Can you work these out from the model? Positions are in its coordinate system, mm. Face numbers are marked on the shaded views. A direction names the side the tool comes from. Give positions to 0.01 mm unless a question says otherwise; leave off trailing zeros. Loops run counter-clockwise (first coordinate to the right, second up) from the corner with the lowest first, then second, coordinate; pieces in that order, holes last. Notation, with made-up numbers: (-28.5, 54.5) -> (11.5, 54.5) arc R17 ccw to (11.5, 71.5) -> close; hole circle Ø1 at (62, 79.5). An arc over 180 degrees is marked (long way). Return JSON: item names as keys, results as strings. Group by question number.
Q1. Suppose I cut it at B-B, the plane y = 0.25. Please give me the cut outline in (x, z).
Q2. Thinking about a two-plate mould opening in X: for the marked faces 3, 4 and 5, which applies, pulls with the +X half, pulls with the -X half, needs draft (parallel to the pull), parting line crosses it, or undercut?
Q3. Suppose I cut it at A-A, the plane z = 0. Please give me the cut outline in (x, y).
Q4. Suppose I cut it at C-C, the plane x = -1.5. Please give me the cut outline in (y, z).
Q5. I need wall thicknesses on line 1 along Y through (x, z) = (0.5, -2.75); line 2 along X through (y, z) = (-8.75, 3). Which ranges of each line are inside material? Lowest first, please. Write a range as [from, to].
Q6. Will these pins go through, and if not, where does the flat tip stop? pin 1 (1.5 mm diameter, centred on x = 2, z = -2, fed in from +Y); pin 2 (1 mm diameter, centred on y = 1, z = 0, fed in from +X); pin 3 (1 mm diameter, centred on y = -3.5, z = -1, fed in from -X).
Q7. Which directions (+Z, -Z, +X, -X, +Y, -Y) give clear straight access to the entire face, cutting with the end or side of a thin tool? Please do the marked faces 1 and 2.
Q8. Suppose I cut it at D-D, the plane z = 1.25. Please give me the cut outline in (x, y), and give its area (3 significant figures).
```python
from build123d import *

# Parameters (mm, degrees)
SKETCH2_R           = 4
BOSS_EXTRUDE1_DEPTH = 15
BOSS_EXTRUDE2_DEPTH = 2


with BuildPart() as part:
    # Sketch2 → Boss-Extrude1 (new body)
    with BuildSketch(Plane(origin=(0, 0, 0), x_dir=(1, 0, 0), z_dir=(0, 1, 0))):
        with Locations(Location((0, 0, 0), (0, 0, 270))):
            Circle(SKETCH2_R)
    extrude(amount=-BOSS_EXTRUDE1_DEPTH)

    # Sketch3 → Boss-Extrude2 (add)
    with BuildSketch(Plane(origin=(0, 0, 0), x_dir=(1, 0, 0), z_dir=(0, 1, 0))):
        with BuildLine():
            Line((-0.75, 2.645751311), (-0.75, -2.645751311))
            ThreePointArc((-0.75, -2.645751311), (-2.75, 0), (-0.75, 2.645751311))
        make_face()
        with BuildLine():
            Line((0.75, 2.645751311), (0.75, -2.645751311))
            ThreePointArc((0.75, -2.645751311), (2.75, 0), (0.75, 2.645751311))
        make_face()
    extrude(amount=BOSS_EXTRUDE2_DEPTH)


solid = part.part
```
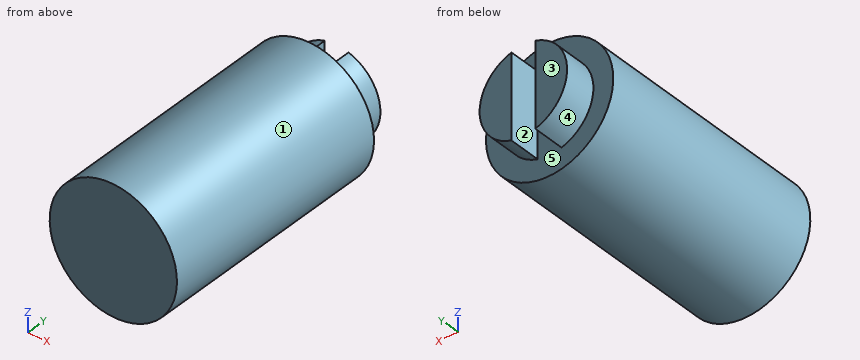
Ans:
{
 "1": {"outline": "(-0.75, -2.65) -> (-0.75, 2.65) arc R2.75 ccw to start; (0.75, -2.65) arc R2.75 ccw to (0.75, 2.65) -> close"},
 "2": {"face 3": "needs draft", "face 4": "pulls with the -X half", "face 5": "undercut"},
 "3": {"outline": "(-4, -15) -> (4, -15) -> (4, 0) -> (2.75, 0) -> (2.75, 2) -> (0.75, 2) -> (0.75, 0) -> (-0.75, 0) -> (-0.75, 2) -> (-2.75, 2) -> (-2.75, 0) -> (-4, 0) -> close"},
 "4": {"outline": "(-15, -3.71) -> (0, -3.71) -> (0, -2.3) -> (2, -2.3) -> (2, 2.3) -> (0, 2.3) -> (0, 3.71) -> (-15, 3.71) -> close"},
 "5": {"line 1": "y = [-15, 0]", "line 2": "x = [-2.65, 2.65]"},
 "6": {"pin 1": "stops at y = 2", "pin 2": "stops at x = 2.75", "pin 3": "stops at x = -3.97"},
 "7": {"face 1": "+Y, -Y", "face 2": "+Z, -Z, +Y"},
 "8": {"outline": "(-3.8, -15) -> (3.8, -15) -> (3.8, 0) -> (2.45, 0) -> (2.45, 2) -> (0.75, 2) -> (0.75, 0) -> (-0.75, 0) -> (-0.75, 2) -> (-2.45, 2) -> (-2.45, 0) -> (-3.8, 0) -> close", "area": "121 mm^2"}
}
